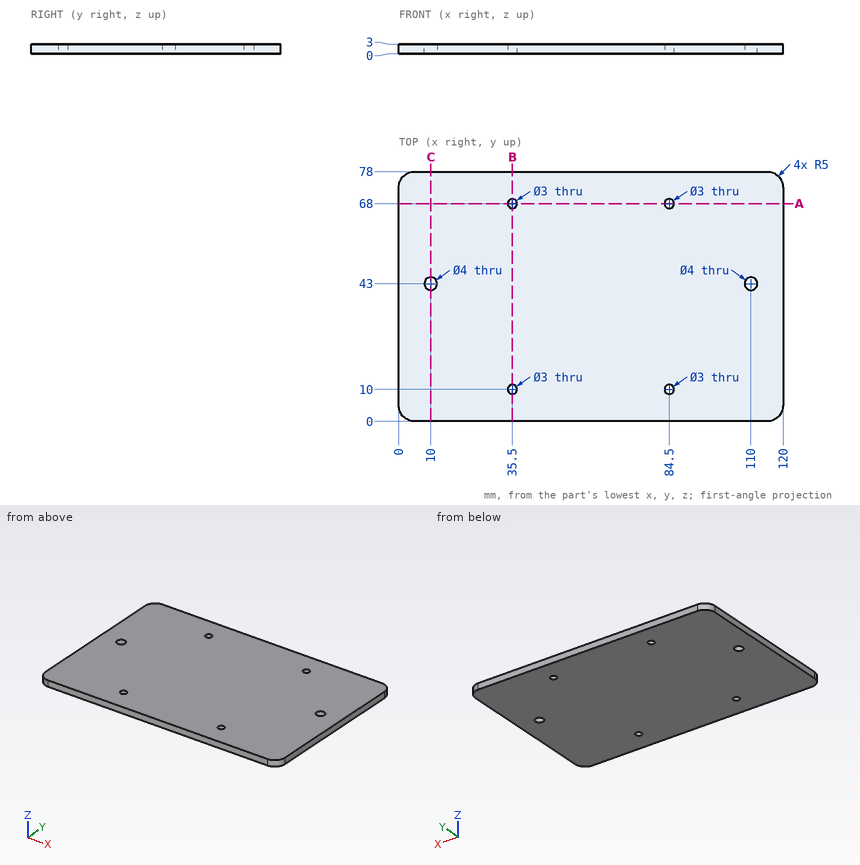
Can you work these out from the drawing? Everything is in mm from the part's minimum corner. Give positions to 0.01 mm unless a question says otherwise; leave off trailing zeros. Order: outer loops, then holes, each group sorted by start corner. A loop starts at its lowest first (then second) coordinate and runs counter-clockwise, first axis right, second up. Notation, with made-up numbers: M 13.5,60.5 L 48.5,60.5 A24 ccw 48.5,70.5 Z; hole C 77,1 d1. An arc over 180 degrees is marked long. Use a Markdown table: item, result. Add a question column.
1. Suppose I cut it at C-C (x = 10). List the corners of the cut face in (y, z) for me.
2. I need wall thicknesses on probe 1 along X at (y, z) = (68, 2); probe 2 along Y at (x, z) = (84.5, 0.75); probe 3 along Y at (x, z) = (10, 1.95). Which ranges of each line are inside material? Lowest first, please. Write a range as from..to.
3. Suppose I cut it at B-B (x = 35.5). List the corners of the cut face in (y, z) for me, and give its area (3 significant figures).
4. Suppose I cut it at A-A (y = 68). List the corners of the cut face in (x, z) for me, and give its area (3 significant figures).
Results list:
| question | item | result |
|---|---|---|
| 1 | outline | M 0,0 L 41,0 L 41,3 L 0,3 Z; M 45,0 L 78,0 L 78,3 L 45,3 Z |
| 2 | probe 1 | x = 0..34, 37..83, 86..120 |
| 2 | probe 2 | y = 0..8.5, 11.5..66.5, 69.5..78 |
| 2 | probe 3 | y = 0..41, 45..78 |
| 3 | outline | M 0,0 L 8.5,0 L 8.5,3 L 0,3 Z; M 11.5,0 L 66.5,0 L 66.5,3 L 11.5,3 Z; M 69.5,0 L 78,0 L 78,3 L 69.5,3 Z |
| 3 | area | 216 mm² |
| 4 | outline | M 0,0 L 34,0 L 34,3 L 0,3 Z; M 37,0 L 83,0 L 83,3 L 37,3 Z; M 86,0 L 120,0 L 120,3 L 86,3 Z |
| 4 | area | 342 mm² |
